Autodesk Inventor part; units mm, degrees
ref_plane "YZ Plane" through (0, 0, 0) normal (1, 0, 0) x (0, 1, 0)
ref_plane "XZ Plane" through (0, 0, 0) normal (0, 1, 0) x (-1, 0, 0)
ref_plane "XY Plane" through (0, 0, 0) normal (0, 0, 1) x (1, 0, 0)
sketch "Sketch1" plane through (0, 0, 0) normal (0, 0, 1) x (1, 0, 0)
  line L0 (-45, 28) -> (45, 28)
  line L1 (45, 28) -> (45, -28)
  line L2 (45, -28) -> (-45, -28)
  line L3 (-45, -28) -> (-45, 28)
  line L4 (-45, 28) -> (45, -28) construction
  line L5 (45, 28) -> (-45, -28) construction
  line L6 (-40, -28) -> (-40, 28)
  circle A0 centre (-36.5, 24.5) radius 1.35
  line L7 (-10.2595, 0) -> (11.3926, 0)
  line L8 (-36.5, 24.5) -> (-7.5, 24.5)
  line L9 (-7.5, 24.5) -> (-7.5, 0)
  circle A1 centre (21.5, 24.5) radius 1.35
  circle A2 centre (-36.5, -24.5) radius 1.35
  circle A3 centre (21.5, -24.5) radius 1.35
  point P0 (0, 0)
  dimension "d0" = 90
  dimension "d1" = 56
  dimension "d4" = 5
  dimension "d5" = 2.7
  dimension "d6" = 3.5
  dimension "d7" = 3.5
  dimension "d8" = 29
  dimension "d9" = 49
extrude "Extrusion1" add sketch "Sketch1" along normal blind 5 contours L0 L1 L2 L6
sketch "Sketch4" plane through (-40, -28, 0) normal (-1, 0, 0) x (0, 0, 1)
  line L0 (0, 0) -> (5, 0)
  line L1 (0, 0) -> (35, 0)
  line L2 (35, 0) -> (35, 56)
  line L3 (35, 56) -> (0, 56)
  line L4 (0, 56) -> (0, 0)
  circle A0 centre (30, 28) radius 1.35
  point P0 (0, 28)
  dimension "d19" = 35
  dimension "d20" = 2.7
  dimension "d21" = 5
  dimension "d22" = 28
  dimension "d25" = 56
extrude "Extrusion3" add sketch "Sketch4" along normal blind 5
fillet "Fillet1" radius 5 1 edges at (-45, 0, 0)
properties part number "Pi4Bracket"
Input: part model. Units: mm. Frame: model coordinates. A direction names the side the tool comes from. Give positions to 0.01 mm unless a question says otherwise; leave off trailing zeros. Order: outer loops, then holes, each group sorted by start corner. A loop starts at its lowest first (then second) coordinate and runs counter-clockwise, first axis right, second up. Notation, with made-up numbers: M 61.25,88 L 80.25,88 A20 cw 80.25,105 Z; hole C 65,11 d10. An arc over 180 degrees is marked long. One line per question, with ' | ' between items. Start each with the question number.
1. Section query D-D (y = 11). Return the cut outline in (x, z).
2. First-contact query: pin 1 Ø2 at (x, y) = (14.5, 14.5) entering from -Z; pin 2 Ø2.5 at (x, y) = (-36.5, 24.5) entering from +Z; pin 3 Ø3.5 at (x, y) = (-36.5, -24.5) entering from +Z. Flat tips, straight axial feed; report the tip coordinate or a pass-through.
3. Section query A-A (x = -36.5). Return the cut outline in (y, z), and give its area (3 significant figures).
4. Section query B-B (z = 30). Return the cut outline in (x, y), and give its area (4 significant figures).
5. Section query C-C (y = 24.5). Return the cut outline in (x, z), and give its area (3 significant figures).
6. Pull-direction query (Z, two-part tool) for faces 3 (the face through (-36.79, -23.18, 2.46)), 4 (the face through (-42.465, -0.406, 31.288)), 5 (the face through (-44, 0, 2)), 6 (the face through (-42, 0, 35)); classes: released by +Z, released by -Z, zero draft, split by the parting line, or undercut.
7. Access query for faces 1 (the face through (-6, -28, 4)), 2 (the face through (-40, 0, 20)). Directions: +Z, -Z, +X, -X, +Y, -Y. A direction counts if a zero-diameter tool reaches every point of the face in a straight line with its end or side. Return the directions, or none.
8. Material intervals for probe 1 along Y at (x, z) = (21.5, 1.1); probe 2 along Y at (x, z) = (-40.95, 30); probe 3 along X at (y, z) = (-24, 3), sorted ascending. Write a range as [from, to].
Here are the results:
1) outline: M -45,5 A5 ccw -40,0 L 45,0 L 45,5 L -40,5 L -40,35 L -45,35 Z
2) pin 1: z = 0 | pin 2: through | pin 3: z = 5
3) outline: M -28,0 L -25.85,0 L -25.85,5 L -28,5 Z; M -23.15,0 L 23.15,0 L 23.15,5 L -23.15,5 Z; M 25.85,0 L 28,0 L 28,5 L 25.85,5 Z | area: 253 mm²
4) outline: M -45,-28 L -40,-28 L -40,-1.35 L -45,-1.35 Z; M -45,1.35 L -40,1.35 L -40,28 L -45,28 Z | area: 266.5 mm²
5) outline: M -45,5 A5 ccw -40,0 L -37.85,0 L -37.85,5 L -40,5 L -40,35 L -45,35 Z; M -35.15,0 L 20.15,0 L 20.15,5 L -35.15,5 Z; M 22.85,0 L 45,0 L 45,5 L 22.85,5 Z | area: 568 mm²
6) face 3: zero draft | face 4: undercut | face 5: released by -Z | face 6: released by +Z
7) face 1: +Z, -Z, +X, -X, -Y | face 2: +Z, +X, +Y, -Y
8) probe 1: [-28, -25.85], [-23.15, 23.15], [25.85, 28] | probe 2: [-28, -1.35], [1.35, 28] | probe 3: [-44.58, -37.75], [-35.25, 20.25], [22.75, 45]
